Autodesk Inventor part; units mm, degrees
ref_plane "YZ Plane" through (0, 0, 0) normal (1, 0, 0) x (0, 1, 0)
ref_plane "XZ Plane" through (0, 0, 0) normal (0, 1, 0) x (-1, 0, 0)
ref_plane "XY Plane" through (0, 0, 0) normal (0, 0, 1) x (1, 0, 0)
sketch "Sketch3" plane through (0, 0, 0) normal (0, 1, 0) x (-1, 0, 0)
  line L0 (0, 0) -> (25, 0)
  line L1 (25, 0) -> (25, -33)
  line L2 (25, -33) -> (0, -33)
  line L3 (0, -33) -> (0, 0)
  dimension "d6" = 25
  dimension "d7" = 33
extrude "Extrusion2" add sketch "Sketch3" along normal blind 3
sketch "Sketch4" plane through (0, 3, 0) normal (0, 1, 0) x (1, 0, 0)
  circle A0 centre (-4, 4) radius 1.5
  line L0 (0, 0) -> (0, 33)
  line L1 (-25, 0) -> (0, 0)
  circle A1 centre (-4, 29) radius 1.5
  line L2 (0, 33) -> (-25, 33)
  circle A2 centre (-20, 4) radius 1.5
  line L3 (-25, 33) -> (-25, 0)
  circle A3 centre (-20, 29) radius 1.5
  dimension "d16" = 3
  dimension "d17" = 4
  dimension "d18" = 4
  dimension "d19" = 3
  dimension "d20" = 4
  dimension "d21" = 4
  dimension "d22" = 3
  dimension "d23" = 16
  dimension "d24" = 4
  dimension "d25" = 5
  dimension "d26" = 3
  dimension "d27" = 4
  dimension "d28" = 16
  dimension "d29" = 25
extrude "Extrusion3" cut sketch "Sketch4" against normal blind 3 contours A0 | A1 | A2 | A3
sketch "Sketch7" plane through (0, 3, 0) normal (0, 1, 0) x (1, 0, 0)
  line L0 (-25, 33) -> (-25, 0)
  line L1 (-25, 0) -> (0, 0)
  line L2 (0, 0) -> (0, -24)
  line L3 (0, -24) -> (-25, -24)
  line L4 (-25, -24) -> (-25, 0)
  dimension "d55" = 24
extrude "Extrusion6" add sketch "Sketch7" against normal blind 3
sketch "Sketch8" plane through (0, 3, 0) normal (0, 1, 0) x (1, 0, 0)
  line L0 (0, -24) -> (-25, -24)
  line L1 (-25, -24) -> (0, -24)
  line L2 (0, -24) -> (0, -21)
  line L3 (0, -21) -> (-25, -21)
  line L4 (-25, -21) -> (-25, -24)
  point P0 (0, 0)
  dimension "d58" = 25
  dimension "d59" = 3
extrude "Extrusion7" add sketch "Sketch8" along normal blind 7
properties part number "CamBracket"
Check sheet for the modelled part. Datum: model origin and axes. Units: mm. A direction names the side the tool comes from. Round coordinates to 2 decimals unless told otherwise and drop trailing zeros. Loops run counter-clockwise (first coordinate to the right, second up) from the corner with the lowest first, then second, coordinate; pieces in that order, holes last.
1. Sectioned sample at B-B on x = -4. Record the boundary of the cut face in (y, z), and give its area (3 significant figures).
2. Sectioned sample at C-C on x = -8.25. Record the boundary of the cut face in (y, z).
3. Sectioned sample at A-A on z = -29. Record the boundary of the cut face in (x, y).
4. Mould release check, pull along Z, two halves, no side actions. Record for faces 3 (the flat face through (-13, 3, -6)), 4 (the flat face through (-13, 1, -33)), 5 (the cylindrical face through (-21.11, 1.52, -30.01)), 6 (the flat face through (-12, 5, 24)): released by +Z, released by -Z, zero draft, split by the parting line, or undercut.
5. Set-up check for faces 1 (the cylindrical face through (-4.195, 1.521, -30.487)), 2 (the flat face through (-12, 6, 21)): record each of +Z, -Z, +X, -X, +Y, -Y from which the full face is reachable in a straight line by a thin tool's end or side.
6. Sectioned sample at D-D on y = 8. Record the boundary of the cut face in (x, z).
7. Gauge pin test, flat ends, axial feed: pin 1 Ø2 at (x, y) = (-13, 8) entering from -Z; pin 2 Ø10 at (x, z) = (-10, -12) entering from +Y. Record the tip position at first contact, or that the pin passes through.
8. Scan lines: probe 1 along X at (y, z) = (1.4, -4); probe 2 along Z at (x, y) = (-4, 1.3); probe 3 along Y at (x, z) = (-4.25, -18). Record each from-to range of solid material in increasing order.
Recorded:
1. outline: (0, -33) - (3, -33) - (3, -30.5) - (0, -30.5) - close; (0, -27.5) - (3, -27.5) - (3, -5.5) - (0, -5.5) - close; (0, -2.5) - (3, -2.5) - (3, 21) - (10, 21) - (10, 24) - (0, 24) - close
1. area: 174 mm2
2. outline: (0, -33) - (3, -33) - (3, 21) - (10, 21) - (10, 24) - (0, 24) - close
3. outline: (-25, 0) - (-21.5, 0) - (-21.5, 3) - (-25, 3) - close; (-18.5, 0) - (-5.5, 0) - (-5.5, 3) - (-18.5, 3) - close; (-2.5, 0) - (0, 0) - (0, 3) - (-2.5, 3) - close
4. face 3: zero draft
4. face 4: released by -Z
4. face 5: undercut
4. face 6: released by +Z
5. face 1: +Y, -Y
5. face 2: -Z, +X, -X, +Y
6. outline: (-25, 21) - (0, 21) - (0, 24) - (-25, 24) - close
7. pin 1: stops at z = 21
7. pin 2: stops at y = 3
8. probe 1: x = -25 to -21.5, -18.5 to -5.5, -2.5 to 0
8. probe 2: z = -33 to -30.5, -27.5 to -5.5, -2.5 to 24
8. probe 3: y = 0 to 3
